from build123d import *

# Parameters (mm, degrees)
EXTRUDE_1_DEPTH           = 2
HOLE_WIZARD_1_D           = 2.8
HOLE_WIZARD_1_DEPTH       = 7.5
HOLE_WIZARD_1_CSINK_D     = 4.8
HOLE_WIZARD_1_CSINK_ANGLE = 90
HOLE_WIZARD_1_TIP         = 0.841204867
SKETCH_4_R                = 5.75
SKETCH_4_R_2              = 4.25
EXTRUDE_1_2_DEPTH         = 0.5
EXTRUDE_2_DEPTH           = 21.5
CHAMFER_1_SIZE            = 2


with BuildPart() as part:
    # 草图1 → Extrude 1 (new body)
    with BuildSketch(Plane.XY):
        with BuildLine():
            Line((-20, -27.9), (0, -27.9))
            ThreePointArc((0, -27.9), (27.9, 0), (0, 27.9))
            Line((0, 27.9), (-20, 27.9))
            ThreePointArc((-20, 27.9), (-47.9, 0), (-20, -27.9))
        make_face()
    extrude(amount=EXTRUDE_1_DEPTH)

    # 打孔尺寸(%根据十字)槽沉头自攻螺钉的类型1
    with Locations(Plane.XY.offset(2)):
        with Locations((-39, 16), (-39, -16), (19, 16), (19, -16), (-60.528138983, 2.67584761), (-55.747291253, 1.462796694)):
            CounterSinkHole(HOLE_WIZARD_1_D / 2, HOLE_WIZARD_1_CSINK_D / 2, depth=HOLE_WIZARD_1_DEPTH, counter_sink_angle=HOLE_WIZARD_1_CSINK_ANGLE)
            with Locations((0, 0, -(HOLE_WIZARD_1_DEPTH + HOLE_WIZARD_1_TIP / 2))):  # 118° drill point
                Cone(0, HOLE_WIZARD_1_D / 2, HOLE_WIZARD_1_TIP, mode=Mode.SUBTRACT)

    # 草图4 → Extrude 1 2 (add)
    # profile 1 of 4: a face of its own
    with BuildSketch(Plane.XY.offset(2)):
        with Locations((11, -19.052558883)):
            Circle(SKETCH_4_R)
        with Locations((11, -19.052558883)):
            Circle(SKETCH_4_R_2, mode=Mode.SUBTRACT)
    # profile 2 of 4: a face of its own
    with BuildSketch(Plane.XY.offset(2)):
        with Locations((11, 19.052558883)):
            Circle(SKETCH_4_R)
        with Locations((11, 19.052558883)):
            Circle(SKETCH_4_R_2, mode=Mode.SUBTRACT)
    # profile 3 of 4: a face of its own
    with BuildSketch(Plane.XY.offset(2)):
        with Locations((-31, 19.052558883)):
            Circle(SKETCH_4_R)
        with Locations((-31, 19.052558883)):
            Circle(SKETCH_4_R_2, mode=Mode.SUBTRACT)
    # profile 4 of 4: a face of its own
    with BuildSketch(Plane.XY.offset(2)):
        with Locations((-31, -19.052558883)):
            Circle(SKETCH_4_R)
        with Locations((-31, -19.052558883)):
            Circle(SKETCH_4_R_2, mode=Mode.SUBTRACT)
    extrude(amount=EXTRUDE_1_2_DEPTH)

    # 草图5 → 拉伸-薄壁2 (add)
    with BuildSketch(Plane.XY.offset(2)):
        with BuildLine():
            ThreePointArc((-38.933849158, 6.442775494), (-31.220488522, 16.55598494), (-18.969199414, 19.973418589))
            Line((-18.969199414, 19.973418589), (-19.098049487, 17.476741266))
            ThreePointArc((-19.098049487, 17.476741266), (-29.817927457, 14.486486822), (-36.567118013, 5.637428557))
            Line((-36.567118013, 5.637428557), (-38.933849158, 6.442775494))
        make_face()
    extrude(amount=-EXTRUDE_2_DEPTH)

    # 倒角1
    chamfer_1_edges = [part.edges().sort_by_distance(p)[0] for p in [
        (-31.220488522, 16.55598494, 0),
        (-29.817927457, 14.486486822, 0),
    ]]
    chamfer(chamfer_1_edges, length=CHAMFER_1_SIZE)


solid = part.part
Model file for the job. Use its own axes, mm. A direction names the side the tool comes from. Give positions to 0.01 mm unless a question says otherwise; leave off trailing zeros. Loops run counter-clockwise (first coordinate to the right, second up) from the corner with the lowest first, then second, coordinate; pieces in that order, holes last.
Item 1: Slice it at D-D (y = 0). Write the cut outline in (x, z), plus the area to 3 significant figures.
Check values:
outline: (-47.9, 0) - (27.9, 0) - (27.9, 2) - (-47.9, 2) - close
area: 152 mm2
Item 2: Drop flat-ended pins along their axis: P1, Ø12, axis at x = -20.5, y = 5, coming from the -Z side; P2, Ø7.5, axis at x = 11, y = 19.05, coming from the +Z side; P3, Ø3.5, axis at x = -39, y = 16, coming from the +Z side. Give the stop position or say it passes through.
Check values:
P1: stops at z = 0
P2: stops at z = 2
P3: stops at z = 1.35
Item 3: Which spindle directions (+Z, -Z, +X, -X, +Y, -Y) get a long thin tool onto all of the face, cutting with end or side? Do faces 5 (the face through (-10, 27.9, 1)), 6 (the face through (-31, -19, 2)). Say none if no direction does.
Check values:
face 5: +Z, -Z, +X, -X, +Y
face 6: +Z
Item 4: Drill centre lines: line 1 along Y through (x, z) = (11, 2.2); line 2 along X through (y, z) = (-16, 0.4); line 3 along Z through (x, y) = (20, -8). Where is each one in solid material? Low to high.
Check values:
line 1: y = -24.8 to -23.3, -14.8 to -13.3, 13.3 to 14.8, 23.3 to 24.8
line 2: x = -42.86 to -40.4, -37.6 to 17.6, 20.4 to 22.86
line 3: z = 0 to 2
Item 5: Mould opens along X. For faces 1 (the face through (-19.03, 18.77, -7.45)), 2 (the face through (-11, 0, 2)), 3 (the face through (11, -19, 2)), 4 (the face through (-30, 15, -19.5)) say: +X half, -X half, draft (parallel to the pull), parting line (faces both ways), or undercut.
Check values:
face 1: +X half
face 2: undercut
face 3: undercut
face 4: draft
Item 6: Slice it at B-B (x = 19). Write the cut outline in (y, z), plus the area to 3 significant figures.
Check values:
outline: (-20.43, 0) - (-17.4, 0) - (-17.4, 1) - (-18.4, 2) - (-20.43, 2) - close; (-14.6, 0) - (14.6, 0) - (14.6, 1) - (13.6, 2) - (-13.6, 2) - (-14.6, 1) - close; (17.4, 0) - (20.43, 0) - (20.43, 2) - (18.4, 2) - (17.4, 1) - close
area: 68.5 mm2
Item 7: Slice it at A-A (x = 11). Write the cut outline in (y, z), plus the area to 3 significant figures.
Check values:
outline: (-25.64, 0) - (25.64, 0) - (25.64, 2) - (24.8, 2) - (24.8, 2.5) - (23.3, 2.5) - (23.3, 2) - (14.8, 2) - (14.8, 2.5) - (13.3, 2.5) - (13.3, 2) - (-13.3, 2) - (-13.3, 2.5) - (-14.8, 2.5) - (-14.8, 2) - (-23.3, 2) - (-23.3, 2.5) - (-24.8, 2.5) - (-24.8, 2) - (-25.64, 2) - close
area: 106 mm2
Item 8: Slice it at C-C (y = -16). Give the number of separate pieces and of enclosed holes in the cut face, plus the area to 3 significant figures.
Check values:
separate pieces: 3
enclosed holes: 0
area: 122 mm2
